from build123d import *

# Parameters (mm, degrees)
F0_W     = 82.8
F0_H     = 65.8
F0_R     = 2.5
F0_W_2   = 8
F0_H_2   = 8
F0_R_2   = 5.5
F0_W_3   = 6.5
F0_H_3   = 6.5
F0_W_4   = 4.5
F0_H_4   = 4.5
F0_R_3   = 1.5
F1_DEPTH = 2
F2_DEPTH = 3
F3_SIZE  = 4


# Not quite as in the source:
# - a feature names something its author has since deleted; it is built from what else it names


with BuildPart() as f1:
    # F0 (on Top) → F1 (new body)
    with BuildSketch(Plane.XY):
        with Locations((0.3088639305, 12.5479439557)):
            Rectangle(F0_W, F0_H)
        with BuildLine():
            ThreePointArc((-37.6911360695, 40.5479439557), (-38.7517962413, 43.1086041274), (-36.1911360695, 42.0479439557))
            Line((-36.1911360695, 42.0479439557), (36.8088639305, 42.0479439557))
            ThreePointArc((36.8088639305, 42.0479439557), (38.3088639305, 43.5479439557), (39.8088639305, 42.0479439557))
            ThreePointArc((39.8088639305, 42.0479439557), (39.3695241023, 40.9872837839), (38.3088639305, 40.5479439557))
            Line((38.3088639305, 40.5479439557), (38.3088639305, -15.4520560443))
            ThreePointArc((38.3088639305, -15.4520560443), (39.3695241023, -15.8913958726), (39.8088639305, -16.9520560443))
            ThreePointArc((39.8088639305, -16.9520560443), (38.3088639305, -18.4520560443), (36.8088639305, -16.9520560443))
            Line((36.8088639305, -16.9520560443), (-36.1911360695, -16.9520560443))
            ThreePointArc((-36.1911360695, -16.9520560443), (-38.7517962413, -18.0127162161), (-37.6911360695, -15.4520560443))
            Line((-37.6911360695, -15.4520560443), (-37.6911360695, 40.5479439557))
        make_face(mode=Mode.SUBTRACT)
        with BuildLine():
            Line((36.8088639305, 42.0479439557), (-36.1911360695, 42.0479439557))
            ThreePointArc((-36.1911360695, 42.0479439557), (-36.6304758977, 40.9872837839), (-37.6911360695, 40.5479439557))
            Line((-37.6911360695, 40.5479439557), (-37.6911360695, -15.4520560443))
            ThreePointArc((-37.6911360695, -15.4520560443), (-36.6304758977, -15.8913958726), (-36.1911360695, -16.9520560443))
            Line((-36.1911360695, -16.9520560443), (36.8088639305, -16.9520560443))
            ThreePointArc((36.8088639305, -16.9520560443), (37.2482037587, -15.8913958726), (38.3088639305, -15.4520560443))
            Line((38.3088639305, -15.4520560443), (38.3088639305, 40.5479439557))
            ThreePointArc((38.3088639305, 40.5479439557), (37.2482037587, 40.9872837839), (36.8088639305, 42.0479439557))
        make_face()
        with BuildLine():
            Line((-35.2911360695, 27.8064392387), (-35.2911360695, 35.4479439557))
            Line((-35.2911360695, 35.4479439557), (-29.4450181015, 35.4479439557))
            ThreePointArc((-29.4450181015, 35.4479439557), (-24.2911360695, 36.6979439557), (-19.1372540375, 35.4479439557))
            Line((-19.1372540375, 35.4479439557), (-8.2911360695, 35.4479439557))
            Line((-8.2911360695, 35.4479439557), (1.2206639384, 35.4479439557))
            ThreePointArc((1.2206639384, 35.4479439557), (3.2088639305, 35.6137958751), (5.1970639225, 35.4479439557))
            Line((5.1970639225, 35.4479439557), (14.7088639305, 35.4479439557))
            Line((14.7088639305, 35.4479439557), (20.7088639305, 35.4479439557))
            Line((20.7088639305, 35.4479439557), (20.7088639305, 36.2488545371))
            Line((20.7088639305, 36.2488545371), (36.7088639305, 36.2488545371))
            Line((36.7088639305, 36.2488545371), (36.7088639305, 15.2488545371))
            Line((36.7088639305, 15.2488545371), (34.7088639305, 15.2488545371))
            Line((34.7088639305, 15.2488545371), (34.7088639305, -14.2511454629))
            Line((34.7088639305, -14.2511454629), (-35.2911360695, -14.5520560443))
            Line((-35.2911360695, -14.5520560443), (-35.2911360695, 23.0894486726))
            ThreePointArc((-35.2911360695, 23.0894486726), (-35.5411360695, 25.4479439557), (-35.2911360695, 27.8064392387))
        make_face(mode=Mode.SUBTRACT)
        with BuildLine():
            Line((-8.2911360695, 35.4479439557), (-19.1372540375, 35.4479439557))
            ThreePointArc((-19.1372540375, 35.4479439557), (-14.6853130215, 31.3037670037), (-13.0411360695, 25.4479439557))
            ThreePointArc((-13.0411360695, 25.4479439557), (-23.105281947, 14.260618538), (-35.2911360695, 23.0894486726))
            Line((-35.2911360695, 23.0894486726), (-35.2911360695, -14.5520560443))
            Line((-35.2911360695, -14.5520560443), (34.7088639305, -14.2511454629))
            Line((34.7088639305, -14.2511454629), (34.7088639305, 15.2488545371))
            Line((34.7088639305, 15.2488545371), (20.7088639305, 15.2488545371))
            Line((20.7088639305, 15.2488545371), (20.7088639305, 35.4479439557))
            Line((20.7088639305, 35.4479439557), (14.7088639305, 35.4479439557))
            Line((14.7088639305, 35.4479439557), (14.7088639305, 27.0416231753))
            ThreePointArc((14.7088639305, 27.0416231753), (15.0832060175, 25.3458466827), (15.2088639305, 23.6137958751))
            ThreePointArc((15.2088639305, 23.6137958751), (15.0832060175, 21.8817450676), (14.7088639305, 20.1859685749))
            Line((14.7088639305, 20.1859685749), (14.7088639305, 12.4479439557))
            Line((14.7088639305, 12.4479439557), (7.604742786, 12.4479439557))
            ThreePointArc((7.604742786, 12.4479439557), (3.2088639305, 11.6137958751), (-1.187014925, 12.4479439557))
            Line((-1.187014925, 12.4479439557), (-8.2911360695, 12.4479439557))
            Line((-8.2911360695, 12.4479439557), (-8.2911360695, 20.1859685749))
            ThreePointArc((-8.2911360695, 20.1859685749), (-8.7911360695, 23.6137958751), (-8.2911360695, 27.0416231753))
            Line((-8.2911360695, 27.0416231753), (-8.2911360695, 35.4479439557))
        make_face()
        with Locations((-5.0911360695, -9.3520560443)):
            Circle(F0_R, mode=Mode.SUBTRACT)
        with Locations((-28.7911360695, -2.5520560443)):
            Circle(F0_R, mode=Mode.SUBTRACT)
        with Locations((-20.7911360695, 4.9479439557)):
            Rectangle(F0_W_2, F0_H_2, mode=Mode.SUBTRACT)
        with Locations((-17.7911360695, -2.5520560443)):
            Circle(F0_R, mode=Mode.SUBTRACT)
        with Locations((5.7088639305, 1.7488545371)):
            Circle(F0_R_2, mode=Mode.SUBTRACT)
        with Locations((27.2088639305, 0.7488545371)):
            Rectangle(F0_W_3, F0_H_3, mode=Mode.SUBTRACT)
        with Locations((5.7088639305, 1.7488545371)):
            Circle(F0_R_2)
        with Locations((5.7088639305, 1.7488545371)):
            Circle(F0_R, mode=Mode.SUBTRACT)
        with BuildLine():
            Line((-26.5411360695, 35.4479439557), (-29.4450181015, 35.4479439557))
            ThreePointArc((-29.4450181015, 35.4479439557), (-33.2261864197, 32.2836864346), (-35.2911360695, 27.8064392387))
            Line((-35.2911360695, 27.8064392387), (-35.2911360695, 23.0894486726))
            ThreePointArc((-35.2911360695, 23.0894486726), (-23.105281947, 14.260618538), (-13.0411360695, 25.4479439557))
            ThreePointArc((-13.0411360695, 25.4479439557), (-14.6853130215, 31.3037670037), (-19.1372540375, 35.4479439557))
            Line((-19.1372540375, 35.4479439557), (-22.0411360695, 35.4479439557))
            ThreePointArc((-22.0411360695, 35.4479439557), (-16.2872307727, 31.8510681931), (-14.0411360695, 25.4479439557))
            ThreePointArc((-14.0411360695, 25.4479439557), (-30.694260307, 17.4440386589), (-26.5411360695, 35.4479439557))
        make_face()
        with Locations((27.2088639305, 0.7488545371)):
            Rectangle(F0_W_3, F0_H_3)
        with Locations((27.2088639305, 0.7488545371)):
            Rectangle(F0_W_4, F0_H_4, mode=Mode.SUBTRACT)
        with BuildLine():
            Line((1.2206639384, 35.4479439557), (-8.2911360695, 35.4479439557))
            Line((-8.2911360695, 35.4479439557), (-8.2911360695, 27.0416231753))
            ThreePointArc((-8.2911360695, 27.0416231753), (-4.7377983891, 32.6054897077), (1.2206639384, 35.4479439557))
        make_face()
        with BuildLine():
            Line((14.7088639305, 35.4479439557), (5.1970639225, 35.4479439557))
            ThreePointArc((5.1970639225, 35.4479439557), (11.1555262501, 32.6054897077), (14.7088639305, 27.0416231753))
            Line((14.7088639305, 27.0416231753), (14.7088639305, 35.4479439557))
        make_face()
        with Locations((-17.7911360695, -2.5520560443)):
            Circle(F0_R)
        with Locations((-17.7911360695, -2.5520560443)):
            Circle(F0_R_3, mode=Mode.SUBTRACT)
        with Locations((-28.7911360695, -2.5520560443)):
            Circle(F0_R)
        with Locations((-28.7911360695, -2.5520560443)):
            Circle(F0_R_3, mode=Mode.SUBTRACT)
        with BuildLine():
            ThreePointArc((-1.187014925, 12.4479439557), (-5.6307626114, 15.4983166779), (-8.2911360695, 20.1859685749))
            Line((-8.2911360695, 20.1859685749), (-8.2911360695, 12.4479439557))
            Line((-8.2911360695, 12.4479439557), (-1.187014925, 12.4479439557))
        make_face()
        with BuildLine():
            Line((14.7088639305, 12.4479439557), (14.7088639305, 20.1859685749))
            ThreePointArc((14.7088639305, 20.1859685749), (12.0484904723, 15.4983166779), (7.604742786, 12.4479439557))
            Line((7.604742786, 12.4479439557), (14.7088639305, 12.4479439557))
        make_face()
        with BuildLine():
            Line((-29.4450181015, 35.4479439557), (-35.2911360695, 35.4479439557))
            Line((-35.2911360695, 35.4479439557), (-35.2911360695, 27.8064392387))
            ThreePointArc((-35.2911360695, 27.8064392387), (-33.2261864197, 32.2836864346), (-29.4450181015, 35.4479439557))
        make_face()
        with BuildLine():
            ThreePointArc((-19.1372540375, 35.4479439557), (-24.2911360695, 36.6979439557), (-29.4450181015, 35.4479439557))
            Line((-29.4450181015, 35.4479439557), (-26.5411360695, 35.4479439557))
            ThreePointArc((-26.5411360695, 35.4479439557), (-24.2911360695, 35.6979439557), (-22.0411360695, 35.4479439557))
            Line((-22.0411360695, 35.4479439557), (-19.1372540375, 35.4479439557))
        make_face()
        with BuildLine():
            Line((-35.2911360695, 23.0894486726), (-35.2911360695, 27.8064392387))
            ThreePointArc((-35.2911360695, 27.8064392387), (-35.5411360695, 25.4479439557), (-35.2911360695, 23.0894486726))
        make_face()
    extrude(amount=F1_DEPTH)

    # F0 (on Top) → F2 (join)
    with BuildSketch(Plane.XY):
        with Locations((27.2088639305, 0.7488545371)):
            Rectangle(F0_W_3, F0_H_3)
        with Locations((27.2088639305, 0.7488545371)):
            Rectangle(F0_W_4, F0_H_4, mode=Mode.SUBTRACT)
        with BuildLine():
            Line((-26.5411360695, 35.4479439557), (-29.4450181015, 35.4479439557))
            ThreePointArc((-29.4450181015, 35.4479439557), (-33.2261864197, 32.2836864346), (-35.2911360695, 27.8064392387))
            Line((-35.2911360695, 27.8064392387), (-35.2911360695, 23.0894486726))
            ThreePointArc((-35.2911360695, 23.0894486726), (-23.105281947, 14.260618538), (-13.0411360695, 25.4479439557))
            ThreePointArc((-13.0411360695, 25.4479439557), (-14.6853130215, 31.3037670037), (-19.1372540375, 35.4479439557))
            Line((-19.1372540375, 35.4479439557), (-22.0411360695, 35.4479439557))
            ThreePointArc((-22.0411360695, 35.4479439557), (-16.2872307727, 31.8510681931), (-14.0411360695, 25.4479439557))
            ThreePointArc((-14.0411360695, 25.4479439557), (-30.694260307, 17.4440386589), (-26.5411360695, 35.4479439557))
        make_face()
        with Locations((-17.7911360695, -2.5520560443)):
            Circle(F0_R)
        with Locations((-17.7911360695, -2.5520560443)):
            Circle(F0_R_3, mode=Mode.SUBTRACT)
        with Locations((5.7088639305, 1.7488545371)):
            Circle(F0_R_2)
        with Locations((5.7088639305, 1.7488545371)):
            Circle(F0_R, mode=Mode.SUBTRACT)
        with BuildLine():
            ThreePointArc((-19.1372540375, 35.4479439557), (-24.2911360695, 36.6979439557), (-29.4450181015, 35.4479439557))
            Line((-29.4450181015, 35.4479439557), (-26.5411360695, 35.4479439557))
            ThreePointArc((-26.5411360695, 35.4479439557), (-24.2911360695, 35.6979439557), (-22.0411360695, 35.4479439557))
            Line((-22.0411360695, 35.4479439557), (-19.1372540375, 35.4479439557))
        make_face()
        with Locations((-28.7911360695, -2.5520560443)):
            Circle(F0_R)
        with Locations((-28.7911360695, -2.5520560443)):
            Circle(F0_R_3, mode=Mode.SUBTRACT)
        with BuildLine():
            Line((-35.2911360695, 23.0894486726), (-35.2911360695, 27.8064392387))
            ThreePointArc((-35.2911360695, 27.8064392387), (-35.5411360695, 25.4479439557), (-35.2911360695, 23.0894486726))
        make_face()
    extrude(amount=-F2_DEPTH)

    # F3
    f3_edges = [f1.edges().sort_by_distance(p)[0] for p in [
        (3.208864, 1.748855, 2),
    ]]
    chamfer(f3_edges, length=F3_SIZE)


solid = f1.part
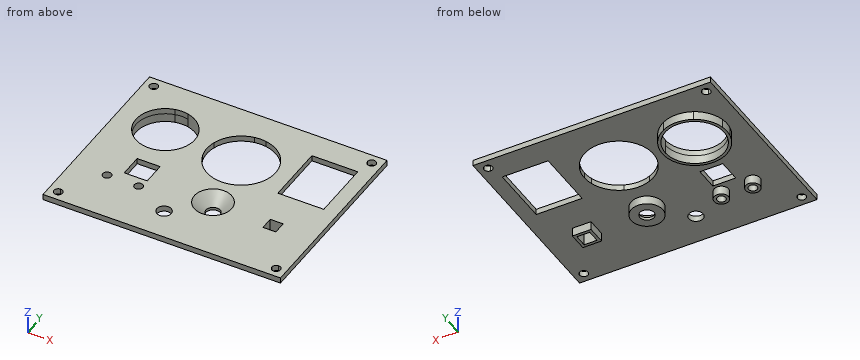
Geometry check sheet. Reference: the model listing, model coordinates, mm. Give positions to 0.01 mm unless a question says otherwise; leave off trailing zeros. Loops run counter-clockwise (first coordinate to the right, second up) from the corner with the lowest first, then second, coordinate; pieces in that order, holes last. Notation, with made-up numbers: M -19.5,34 L 0.5,34 A16 ccw 0.5,42 Z; hole C 56.25,-15 d9. An arc over 180 degrees is marked long. Write each question's results on one line, items separated by ' | '.
1) Section check C-C, the plane y = 10. Record the boundary of the cut face in (x, z).
Answers follow:
outline: M -41.09,0 L 41.71,0 L 41.71,2 L -41.09,2 Z
2) Section check D-D, the plane y = 33. Record the boundary of the cut face in (x, z), plus the area to 3 significant figures.
Answers follow:
outline: M -41.09,0 L -32.63,0 L -32.63,-3 L -31.22,-3 L -31.22,2 L -41.09,2 Z; M -17.36,-3 L -15.95,-3 L -15.95,0 L -4.27,0 L -4.27,2 L -17.36,2 Z; M 10.69,0 L 20.71,0 L 20.71,2 L 10.69,2 Z; M 36.71,0 L 41.71,0 L 41.71,2 L 36.71,2 Z | area: 84.4 mm2
3) Thickness scan on line 1 (Y direction, x = 25.5, z = 0.65); line 2 (Y direction, x = 28.5, z = -0.7); line 3 (X direction, y = 0, z = -1.2). Record the ranges inside material, lowest first.
Answers follow:
line 1: -20.35 to -1.5, 3 to 15.25, 36.25 to 45.45 | line 2: -2.5 to -1.5, 3 to 4 | line 3: 0.49 to 2.91, 8.51 to 10.92, 23.96 to 24.96, 29.46 to 30.46
4) Section check A-A, the plane z = -0.75. Count the separate pieces of the cut face and the enclosed holes in it, plus the area to 3 significant figures.
Answers follow:
separate pieces: 5 | enclosed holes: 5 | area: 166 mm2
5) Section check B-B, the plane y = 22. Record the boundary of the cut face in (x, z), plus the area to 3 significant figures.
Answers follow:
outline: M -41.09,0 L -35,0 L -35,-3 L -33.94,-3 L -33.94,2 L -41.09,2 Z; M -14.64,-3 L -13.58,-3 L -13.58,0 L -8.68,0 L -8.68,2 L -14.64,2 Z; M 15.1,0 L 20.71,0 L 20.71,2 L 15.1,2 Z; M 36.71,0 L 41.71,0 L 41.71,2 L 36.71,2 Z | area: 53.8 mm2
6) Gauge pin test, flat ends, axial feed: pin 1 (2 mm diameter, centred on y = 0, z = -2, fed in from -X); pin 2 (1 mm diameter, centred on x = 26.5, z = -1.5, fed in from +Y); pin 3 (6.5 mm diameter, centred on x = 5.71, y = 1.75, fed in from +Z). Record the tip position at first contact, or that the pin passes through.
Answers follow:
pin 1: x = -30.75 | pin 2: y = 4 | pin 3: z = -1.25
